Build history of the part. All positions in model axes, mm. A direction names the side the tool comes from. Coordinates: 2 decimals unless noted, no trailing zeros. Loops run counter-clockwise (first coordinate to the right, second up) from the corner with the lowest first, then second, coordinate; pieces in that order, holes last.
(1) Flat gauge pins, fed straight in: P1, Ø2, axis at x = 119.5, y = -16.5, coming from the +Z side; P2, Ø6, axis at y = -43, z = 45.5, coming from the -X side; P3, Ø8, axis at x = 11, z = 87.5, coming from the -Y side; P4, Ø10, axis at x = 92.5, y = -46.5, coming from the -Z side. Where does each tip first touch, or does it go through?
(2) Slice it at B-B (x = 15). Give the cut face in (y, z), and give its area (4 significant figures).
(3) Wall check: L1, parallel to Y at x = 20.5, z = 64; L2, parallel to Y at x = 42, z = 68; L3, parallel to Y at x = 16, z = 89. Give the ranges that are in metal, low to high.
(4) Slice it at C-C (z = 19.5). Give the cut face in (x, y).
(5) Two-plate mould, pull along X, no slides. Class faces 1 (the face through (79.964, -35.921, 46.262)), 2 (the face through (138.798, 4.299, 5.07)), 3 (the face through (-4.445, -53.944, 5.07)): pulls with the +X half, pulls with the -X half, needs draft (parallel to the pull), parting line crosses it, or undercut.
(6) Slice it at D-D (x = 50). Give the cut face in (y, z), and give its area (3 significant figures).
(7) Tool access for faces 4 (the face through (138.8, -53.99, 5.07)), 5 (the face through (105.117, -16, 63)): list every direction of +Z, -Z, +X, -X, +Y, -Y with a clear straight run to the whole face (end or side of a thin tool).
from build123d import *

# Parameters (mm, degrees)
F0_W     = 135
F0_H     = 100
F1_DEPTH = 50
F2_W     = 12
F2_H     = 7
F2_W_2   = 9
F3_DEPTH = 75
F5_D     = 7
F5_DEPTH = 52
F5_TIP   = 2.1030121666
F6_W     = 145
F6_H     = 60
F7_DEPTH = 10
F8_R     = 7
F9_R     = 3


# Not quite as in the source:
# - a feature names something its author has since deleted; it is built from what else it names


with BuildPart() as f1:
    # F0 (on Front) → F1 (new body)
    with BuildSketch(Plane.XZ):
        with Locations((67.5, 50)):
            Rectangle(F0_W, F0_H)
    extrude(amount=F1_DEPTH)

    # F2 (on face) → F3 (cut)
    with BuildSketch(Plane.XY.offset(100)):
        with Locations((19.1170862466, -16.0328453556)):
            Rectangle(F2_W, F2_H)
        with Locations((39.1170862466, -16.0328453556)):
            Rectangle(F2_W, F2_H)
        with Locations((59.1170862466, -16.0328453556)):
            Rectangle(F2_W, F2_H)
        with Locations((79.1170862466, -16.0328453556)):
            Rectangle(F2_W, F2_H)
        with Locations((99.1170862466, -16.0328453556)):
            Rectangle(F2_W, F2_H)
        with Locations((119.5874011219, -15.8250607699)):
            Rectangle(F2_W_2, F2_H)
    extrude(amount=-F3_DEPTH, mode=Mode.SUBTRACT)

    # F5
    with Locations(Plane.XY.offset(100)):
        with Locations((20.5715699643, -35.9477512538), (40.5715699643, -35.9477512538), (60.5715699643, -35.9477512538), (80.5715699643, -35.9477512538), (100.5715699643, -35.9477512538), (120.5715699643, -35.9477512538)):
            Hole(F5_D / 2, depth=F5_DEPTH)
            with Locations((0, 0, -(F5_DEPTH + F5_TIP / 2))):  # 118° drill point
                Cone(0, F5_D / 2, F5_TIP, mode=Mode.SUBTRACT)

    # F6 (on Top) → F7 (join)
    with BuildSketch(Plane.XY):
        with Locations((67.1998835728, -24.8457092833)):
            Rectangle(F6_W, F6_H)
    extrude(amount=F7_DEPTH)

    # F8
    f8_edges = [f1.edges().sort_by_distance(p)[0] for p in [
        (0, -50, 55),
        (135, -50, 55),
        (135, 0, 55),
        (0, 0, 55),
    ]]
    fillet(f8_edges, radius=F8_R)

    # F9
    f9_edges = [f1.edges().sort_by_distance(p)[0] for p in [
        (-5.300116, 5.154291, 5),
        (-5.300116, -54.845709, 5),
        (139.699884, -54.845709, 5),
        (139.699884, 5.154291, 5),
    ]]
    fillet(f9_edges, radius=F9_R)


solid = f1.part
Response values:
1. P1: stops at z = 25
1. P2: stops at x = 0
1. P3: stops at y = -50
1. P4: stops at z = 0
2. outline: (-54.85, 0) - (5.15, 0) - (5.15, 10) - (0, 10) - (0, 100) - (-12.53, 100) - (-12.53, 25) - (-19.53, 25) - (-19.53, 100) - (-50, 100) - (-50, 10) - (-54.85, 10) - close
2. area: 4,575 mm2
3. L1: y = -50 to -39.45, -32.45 to -19.53, -12.53 to 0
3. L2: y = -50 to -39.14, -32.75 to -19.53, -12.53 to 0
3. L3: y = -50 to -19.53, -12.53 to 0
4. outline: (0, -43) arc R7 ccw to (7, -50) - (128, -50) arc R7 ccw to (135, -43) - (135, -7) arc R7 ccw to (128, 0) - (7, 0) arc R7 ccw to (0, -7) - close
5. face 1: undercut
5. face 2: pulls with the +X half
5. face 3: pulls with the -X half
6. outline: (-54.85, 0) - (5.15, 0) - (5.15, 10) - (0, 10) - (0, 100) - (-50, 100) - (-50, 10) - (-54.85, 10) - close
6. area: 5,100 mm2
7. face 4: +Z, -Z, +X, -Y
7. face 5: +Z
